Can you work these out from the model? Positions are in its coordinate system, mm. Give positions to 0.01 mm unless a question says otherwise; leave off trailing zeros. Write each loop counter-clockwise with the first axis right and the second up, starting at its lowest first coordinate (ties: lowest second). Pieces come first, ordered by that corner, then holes. Notation, with made-up numbers: (-32, -23.75) - (-7, -23.75) arc R16 ccw to (-7, -16.75) - close; hole circle Ø5 at (74, 47). An arc over 180 degrees is marked (long way). Use a Markdown table: item, result. Add a question column.
```python
from build123d import *


with BuildPart() as f2:
    # F1 (on Right) → F2 (revolve)
    with BuildSketch(Plane.YZ):
        with BuildLine():
            Line((-5.299645, 0.014583), (-5, 0))
            ThreePointArc((-5, 0), (-11.414984, 52.575505), (-35, 100))
            Line((-35, 100), (-35.242136, 99.822883))
            ThreePointArc((-35.242136, 99.822883), (-11.702331, 52.489301), (-5.299645, 0.014583))
        make_face()
    revolve(axis=Axis((0, 0, 50), (0, 0, 1)))

    # F1 (on Right) → F3 (revolve)
    with BuildSketch(Plane.YZ):
        Polygon((34.6, 100.25), (34.6, 100), (34.6, 99.75), (35.4, 99.75), (35.4, 100.25), align=None)
    revolve(axis=Axis((0, 0, 50), (0, 0, 1)))


solid = f2.part
```
Q1. If I drill on probe 1 along Y at (x, z) = (0, 100); probe 2 along X at (y, z) = (-2, 37), over which ranges is the centre line in solid material (lowest first)? Write a range as [from, to].
Q2. I'm going to push flat-ended pins straight in: P1, Ø8, axis at y = -5.5, z = 82, coming from the -X side; P2, Ø4, axis at y = 8, z = 30.5, coming from the +X side; P3, Ø6, axis at x = 8, y = 16, coming from the +Z side. Where does each tip first touch, or does it pass through?
Q3. Suppose I cut it at D-D (z = 73). Please give me the cut outline in (x, y), and give its area (3 significant figures).
Q4. Suppose I cut it at C-C (z = 45). Please give me the cut outline in (x, y), and give its area (3 significant figures).
Q5. If we mould it in two halves opening along X, with no side actions, what happens to faces 1 (the cylindrical face through (-10.4, 33, 100)), 2 (the flat face through (34, 8, 100.25)), 3 (the cylindrical face through (-10.633, 33.765, 100.004))? For each: released by +X, released by -X, zero draft, split by the parting line, or undercut.
Derived:
| question | item | result |
|---|---|---|
| 1 | probe 1 | [-35.4, -34.6], [34.6, 35.4] |
| 1 | probe 2 | [-7.65, -7.33], [7.33, 7.65] |
| 2 | P1 | x = -25.75 |
| 2 | P2 | x = 3.26 |
| 2 | P3 | z = 76.69 |
| 3 | outline | circle Ø38.93 at (0, 0); hole circle Ø38.27 at (0, 0) |
| 3 | area | 40.0 mm² |
| 4 | outline | circle Ø19.31 at (0, 0); hole circle Ø18.7 at (0, 0) |
| 4 | area | 18.4 mm² |
| 5 | face 1 | undercut |
| 5 | face 2 | zero draft |
| 5 | face 3 | split by the parting line |
